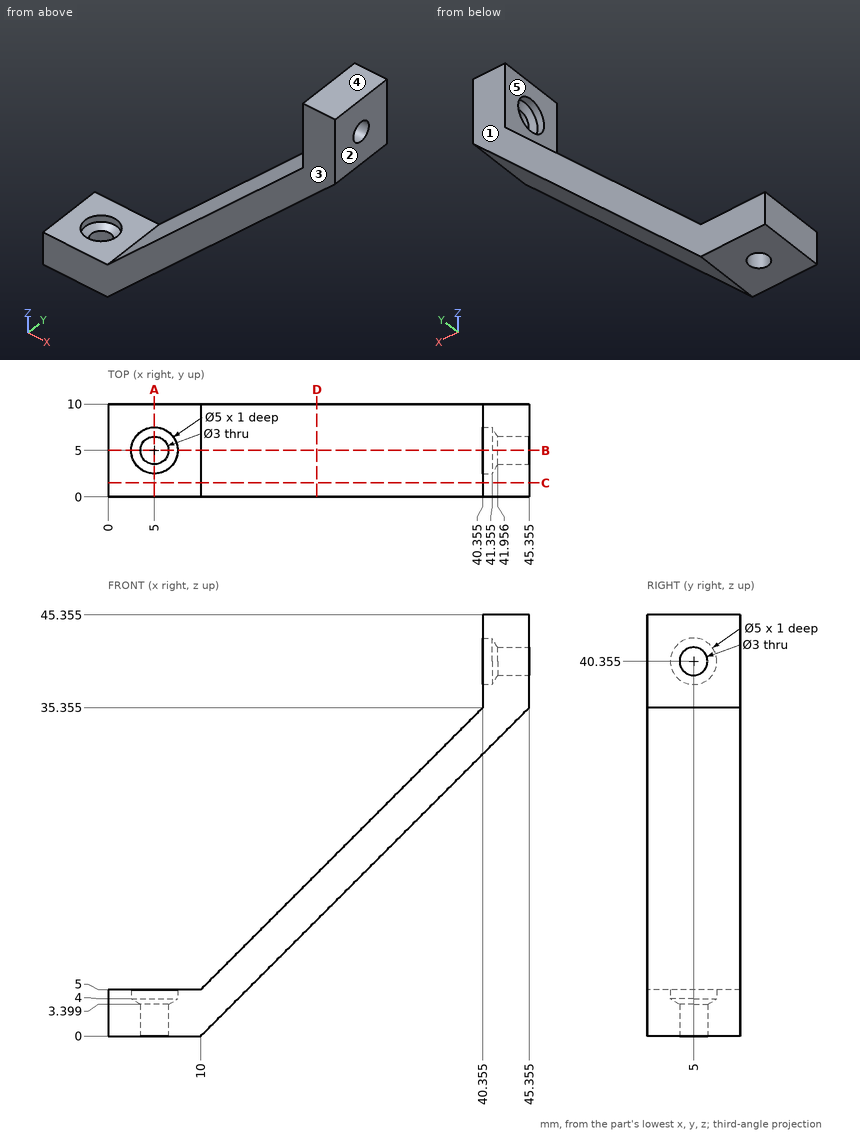
Geometry: see drawing. Coordinates: mm, zero at the bounding-box minimum. A direction names the side the tool comes from. Give positions to 0.01 mm unless a question says otherwise; leave off trailing zeros. Write each loop counter-clockwise with the first axis right and the second up, starting at its lowest first coordinate (ties: lowest second). Pieces come first, ordered by that corner, then holes. Notation, with made-up numbers: (88, 52.25) - (129, 52.25) arc R13 ccw to (129, 65.25) - close; hole circle Ø11 at (-24, 3). An arc over 180 degrees is marked (long way). Return JSON: item names as keys, results as strings. Group by question number.
1) Section C-C on y = 1.5. Return the cut outline in (x, z) (1 decimal).
2) Section D-D on x = 22.5. Return the cut outline in (y, z).
3) Line query: line 1 (Z direction, x = 43, y = 5) (1 decimal); line 2 (X direction, y = 5, z = 1.8); line 3 (Z direction, x = 6.5, y = 9). Output: solid intervals per line, ascending.
4) First-contact query: P1, Ø4, axis at x = 5, y = 5, coming from the +Z side; P2, Ø1.5, axis at y = 4, z = 16.5, coming from the -X side; P3, Ø1.5, axis at y = 6.5, z = 20.5, coming from the +X side. Flat tips, straight axial feed; report the tip coordinate or a pass-through.
5) Section B-B on y = 5. Return the cut outline in (x, z) (1 decimal).
6) Mould query, pull axis Y, two halves, no side actions, for the marked faces 1, 2 and 3. Classes: released by +Y, released by -Y, zero draft, split by the parting line, or undercut.
7) Set-up query: the marked faces 4 and 5. Return all of +Z, -Z, +X, -X, +Y, -Y with unobstructed straight access to the full face (end or side cutting, diameter ignored); none if empty.
8) Section A-A on x = 5. Return the cut outline in (y, z), plus the area to 3 significant figures.
Filled in:
{
 "1": {"outline": "(0, 0) - (10, 0) - (45.4, 35.4) - (45.4, 45.4) - (40.4, 45.4) - (40.4, 35.4) - (10, 5) - (0, 5) - close"},
 "2": {"outline": "(0, 12.5) - (10, 12.5) - (10, 17.5) - (0, 17.5) - close"},
 "3": {"line 1": "z = 33 to 38.9, 41.9 to 45.4", "line 2": "x = 0 to 3.5, 6.5 to 11.8", "line 3": "z = 0 to 5"},
 "4": {"P1": "stops at z = 3.7", "P2": "stops at x = 20.75", "P3": "stops at x = 31.25"},
 "5": {"outline": "(0, 0) - (3.5, 0) - (3.5, 3.4) - (2.5, 4) - (2.5, 5) - (0, 5) - close; (6.5, 0) - (10, 0) - (45.4, 35.4) - (45.4, 38.9) - (42, 38.9) - (41.4, 37.9) - (40.4, 37.9) - (40.4, 35.4) - (10, 5) - (7.5, 5) - (7.5, 4) - (6.5, 3.4) - close; (40.4, 42.9) - (41.4, 42.9) - (42, 41.9) - (45.4, 41.9) - (45.4, 45.4) - (40.4, 45.4) - close"},
 "6": {"face 1": "released by +Y", "face 2": "zero draft", "face 3": "released by -Y"},
 "7": {"face 4": "+Z, +X, -X, +Y, -Y", "face 5": "+Z, -X, +Y, -Y"},
 "8": {"outline": "(0, 0) - (3.5, 0) - (3.5, 3.4) - (2.5, 4) - (2.5, 5) - (0, 5) - close; (6.5, 0) - (10, 0) - (10, 5) - (7.5, 5) - (7.5, 4) - (6.5, 3.4) - close", "area": "32.4 mm^2"}
}
